from build123d import *

# Parameters (mm, degrees)
CUT_EXTRUDE1_REACH       = 144.018
BOSS_EXTRUDE1_DEPTH      = 150
BOSS_EXTRUDE1_DEPTH_BACK = 30
SKETCH3_R                = 8


with BuildPart() as part:
    # Sketch1 → Revolve2 (revolve)
    with BuildSketch(Plane.XY, mode=Mode.PRIVATE) as revolve2_sk:
        with BuildLine():
            Line((8, 8), (8, -8))
            Line((8, -8), (14, -8))
            Line((14, -8), (14, -5))
            Line((14, -5), (94, -5))
            Line((94, -5), (94, -8))
            Line((94, -8), (100, -8))
            Line((100, -8), (100, -4))
            ThreePointArc((100, -4), (96, 0), (100, 4))
            Line((100, 4), (100, 8))
            Line((100, 8), (94, 8))
            Line((94, 8), (94, 5))
            Line((94, 5), (14, 5))
            Line((14, 5), (14, 8))
            Line((14, 8), (14, 18))
            Line((14, 18), (8, 18))
            Line((8, 18), (8, 8))
        make_face()
    revolve(revolve2_sk.sketch.rotate(Axis((0, 60.317614973, 0), (0, -1, 0)), 90), axis=Axis((0, 60.317614973, 0), (0, -1, 0)))

    # Cut-Extrude1: up to this face of the body (flat: up to its plane)
    cut_extrude1_end = Plane(part.part.faces().sort_by_distance((0, -5, -16.658721497))[0])
    # Sketch2 → Cut-Extrude1 (cut, up to the picked face)
    with BuildSketch(Plane(origin=(0, 5, 0), x_dir=(1, 0, 0), z_dir=(0, 1, 0)), mode=Mode.PRIVATE) as cut_extrude1_sk1:
        with BuildLine():
            Line((14, 14), (14, 173.435867109))
            ThreePointArc((14, 173.435867109), (123.036579926, 123.036579926), (173.435867109, 14))
            Line((173.435867109, 14), (14, 14))
        make_face()
    cut_extrude1_tool1 = split(extrude(cut_extrude1_sk1.sketch, amount=-CUT_EXTRUDE1_REACH, mode=Mode.PRIVATE), bisect_by=cut_extrude1_end, keep=Keep.BOTH, mode=Mode.PRIVATE)
    # Sketch2 → Cut-Extrude1 (cut, up to the picked face)
    with BuildSketch(Plane(origin=(0, 5, 0), x_dir=(1, 0, 0), z_dir=(0, 1, 0)), mode=Mode.PRIVATE) as cut_extrude1_sk2:
        with BuildLine():
            Line((-173.435867109, -14), (-14, -14))
            Line((-14, -14), (-14, -173.435867109))
            ThreePointArc((-14, -173.435867109), (-123.036579926, -123.036579926), (-173.435867109, -14))
        make_face()
    cut_extrude1_tool2 = split(extrude(cut_extrude1_sk2.sketch, amount=-CUT_EXTRUDE1_REACH, mode=Mode.PRIVATE), bisect_by=cut_extrude1_end, keep=Keep.BOTH, mode=Mode.PRIVATE)
    # Sketch2 → Cut-Extrude1 (cut, up to the picked face)
    with BuildSketch(Plane(origin=(0, 5, 0), x_dir=(1, 0, 0), z_dir=(0, 1, 0)), mode=Mode.PRIVATE) as cut_extrude1_sk3:
        with BuildLine():
            Line((-14, 14), (-14, 173.435867109))
            ThreePointArc((-14, 173.435867109), (-123.036579926, 123.036579926), (-173.435867109, 14))
            Line((-173.435867109, 14), (-14, 14))
        make_face()
    cut_extrude1_tool3 = split(extrude(cut_extrude1_sk3.sketch, amount=-CUT_EXTRUDE1_REACH, mode=Mode.PRIVATE), bisect_by=cut_extrude1_end, keep=Keep.BOTH, mode=Mode.PRIVATE)
    # Sketch2 → Cut-Extrude1 (cut, up to the picked face)
    with BuildSketch(Plane(origin=(0, 5, 0), x_dir=(1, 0, 0), z_dir=(0, 1, 0)), mode=Mode.PRIVATE) as cut_extrude1_sk4:
        with BuildLine():
            Line((14, -14), (173.435867109, -14))
            ThreePointArc((173.435867109, -14), (123.036579926, -123.036579926), (14, -173.435867109))
            Line((14, -173.435867109), (14, -14))
        make_face()
    cut_extrude1_tool4 = split(extrude(cut_extrude1_sk4.sketch, amount=-CUT_EXTRUDE1_REACH, mode=Mode.PRIVATE), bisect_by=cut_extrude1_end, keep=Keep.BOTH, mode=Mode.PRIVATE)
    add(cut_extrude1_tool1.solids().sort_by(Axis((80.012708, 5, -80.012708), (0, -1, 0)))[0], mode=Mode.SUBTRACT)
    add(cut_extrude1_tool2.solids().sort_by(Axis((-80.012708, 5, 80.012708), (0, -1, 0)))[0], mode=Mode.SUBTRACT)
    add(cut_extrude1_tool3.solids().sort_by(Axis((-80.012708, 5, -80.012708), (0, -1, 0)))[0], mode=Mode.SUBTRACT)
    add(cut_extrude1_tool4.solids().sort_by(Axis((80.012708, 5, 80.012708), (0, -1, 0)))[0], mode=Mode.SUBTRACT)

    # Sketch3 → Boss-Extrude1 (add, two sides: drawn at the far end of the back side and taken through both)
    with BuildSketch(Plane.XZ.offset(8).offset(-BOSS_EXTRUDE1_DEPTH_BACK)):
        with Locations(Location((0, 0, 0), (0, 0, 270))):
            Circle(SKETCH3_R)
    extrude(amount=BOSS_EXTRUDE1_DEPTH + BOSS_EXTRUDE1_DEPTH_BACK)


solid = part.part
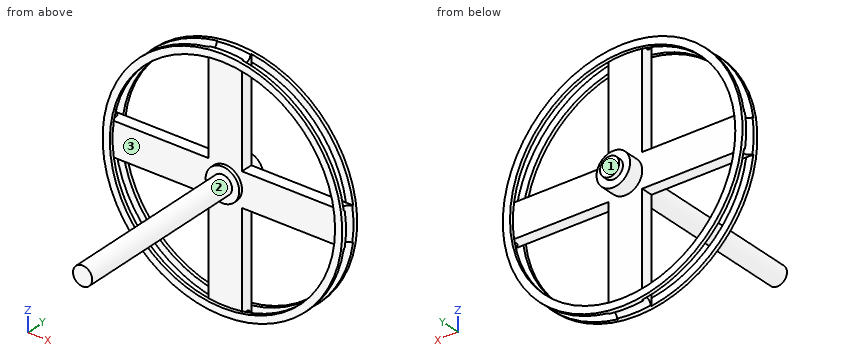
The listing builds one solid part. Answer for the finished solid, in the listing's coordinates (mm). Face numbers are marked on the shaded views. Coordinates: 2 decimals unless noted, no trailing zeros. Loops run counter-clockwise (first coordinate to the right, second up) from the corner with the lowest first, then second, coordinate; pieces in that order, holes last.
1) Find section A-A on x = -48. Write down the section's boundary in (y, z).
2) Find the intervals of material crossed by L1, parallel to X at y = -6.9, z = 0; L2, parallel to Y at x = -37.5, z = -2; L3, parallel to X at y = 7, z = 66, in increasing order.
3) Determine the mould class of the marked faces 1, 2 and 3 for opening direction X: pulls with the +X half, pulls with the -X half, needs draft (parallel to the pull), parting line crosses it, or undercut.
4) Find section B-B on z = 62. Write down the section's boundary in (x, y).
5) Find section D-D on y = -75. Write down the section's boundary in (x, z), then the cut area to 3 significant figures.
6) Flat-ended cylindrical pins translate along their axes: pin 1 Ø3 at (x, y) = (-39.5, 1.5) entering from +Z; pin 2 Ø11 at (x, y) = (-43, -2.5) entering from -Z; pin 3 Ø11 at (x, y) = (40, 0.5) entering from -Z. Find the tip coordinate at first contact, or state that the pin passes through.
Values:
1. outline: (-8, -87.73) - (-5, -87.73) - (-5, -80.82) - (-8, -80.82) - close; (-8, 80.82) - (-5, 80.82) - (-5, 87.73) - (-8, 87.73) - close; (-5, -14) - (5, -14) - (5, 14) - (-5, 14) - close; (5, -87.73) - (8, -87.73) - (8, -80.82) - (5, -80.82) - close; (5, 80.82) - (8, 80.82) - (8, 87.73) - (5, 87.73) - close
2. L1: x = -100 to -94, -14 to 14, 94 to 100
2. L2: y = -5 to 5
2. L3: x = -75.13 to -66.93, 66.93 to 75.13
3. face 1: needs draft
3. face 2: parting line crosses it
3. face 3: undercut
4. outline: (-78.46, -8) - (-70.65, -8) - (-70.65, -5) - (-78.46, -5) - close; (-78.46, 5) - (-70.65, 5) - (-70.65, 8) - (-78.46, 8) - close; (-14, -5) - (14, -5) - (14, 5) - (-14, 5) - close; (70.65, -8) - (78.46, -8) - (78.46, -5) - (70.65, -5) - close; (70.65, 5) - (78.46, 5) - (78.46, 8) - (70.65, 8) - close
5. outline: circle Ø16 at (0, 0)
5. area: 201 mm2
6. pin 1: stops at z = 14
6. pin 2: stops at z = -92.46
6. pin 3: stops at z = -92.97
